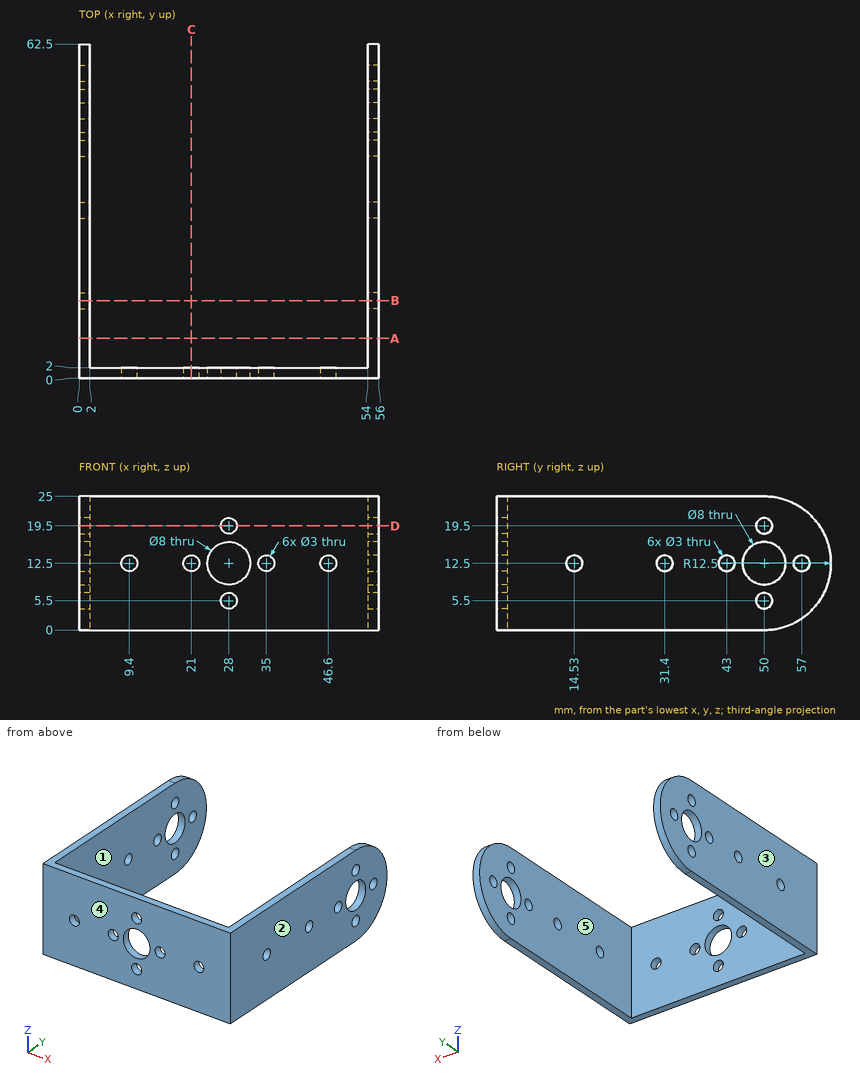
The drawing under review shows one solid part. Ordinate dimensions are in mm from its lowest x, y, z. A direction names the side the tool comes from. Round coordinates to 2 decimals unless told otherwise and drop trailing zeros. Write each loop counter-clockwise with the first axis right and the second up, starting at its lowest first coordinate (ties: lowest second). Pieces come first, ordered by that corner, then holes. Notation, with made-up numbers: (-10.75, 10.5) - (14.25, 10.5) arc R16 cw to (14.25, 40.5) - close; hole circle Ø8 at (43.5, 85). An arc over 180 degrees is marked (long way). Use one line per item in the form item = value.
Q1. Tool access review of the marked faces 1 and 2: name each direction out of +Z, -Z, +X, -X, +Y, -Y from which nothing blocks a thin tool from reaching the whole face with its end or side.
Answer key:
face_1 = +Z, -Z, +Y
face_2 = +Z, -Z, +X, +Y, -Y
Q2. Consider section B-B (y = 14.53). State the section outline as (x, z) points.
Answer key:
outline = (0, 0) - (2, 0) - (2, 11) - (0, 11) - close; (0, 14) - (2, 14) - (2, 25) - (0, 25) - close; (54, 0) - (56, 0) - (56, 11) - (54, 11) - close; (54, 14) - (56, 14) - (56, 25) - (54, 25) - close
Q3. Consider section D-D (z = 19.5). State the section outline as (x, y) points.
Answer key:
outline = (0, 0) - (26.5, 0) - (26.5, 2) - (2, 2) - (2, 48.5) - (0, 48.5) - close; (0, 51.5) - (2, 51.5) - (2, 60.36) - (0, 60.36) - close; (29.5, 0) - (56, 0) - (56, 48.5) - (54, 48.5) - (54, 2) - (29.5, 2) - close; (54, 51.5) - (56, 51.5) - (56, 60.36) - (54, 60.36) - close
Q4. Consider section C-C (x = 21). State the section outline as (y, z) points, and give its area (3 significant figures).
Answer key:
outline = (0, 0) - (2, 0) - (2, 11) - (0, 11) - close; (0, 14) - (2, 14) - (2, 25) - (0, 25) - close
area = 44.0 mm2
Q5. For line 1 (Y direction, x = 55, z = 12.5); line 2 (Z direction, x = 28, y = 1.2); line 3 (X direction, y = 7.5, z = 9), list the stretches that pass through material, from the lowest coordinate up. Write a range as [from, to].
Answer key:
line_1 = [0, 13.03], [16.03, 29.9], [32.9, 41.5], [44.5, 46], [54, 55.5], [58.5, 62.5]
line_2 = [0, 4], [7, 8.5], [16.5, 18], [21, 25]
line_3 = [0, 2], [54, 56]
Q6. Draft analysis for pull direction X (two halves, no side actions). For the marked faces 3, 4 and 5, state which applies: +X half, -X half, draft (parallel to the pull), parting line (faces both ways), or undercut.
Answer key:
face_3 = -X half
face_4 = draft
face_5 = undercut
Q7. Consider section A-A (y = 7.5). State the section outline as (x, z) points, and give its area (3 significant figures).
Answer key:
outline = (0, 0) - (2, 0) - (2, 25) - (0, 25) - close; (54, 0) - (56, 0) - (56, 25) - (54, 25) - close
area = 100 mm2
Q8. Insertion check: pin 1 Ø3.5 at (x, z) = (9.4, 12.5) entering from +Y. The pin has a flat end and moves straight along its axis. Give the tip position at first contact, or say it passes through.
Answer key:
pin_1 = 2
